Build history of the part. All positions in model axes, mm. Face numbers are marked on the shaded views. Round coordinates to 2 decimals unless told otherwise and drop trailing zeros. Loops run counter-clockwise (first coordinate to the right, second up) from the corner with the lowest first, then second, coordinate; pieces in that order, holes last. Notation, with made-up numbers: M -5,33 L 30,33 A24 ccw 30,62 Z; hole C 12.25,-28.5 d1. An arc over 180 degrees is marked long. Use one line per item in the form item = value. Start each with the question number.
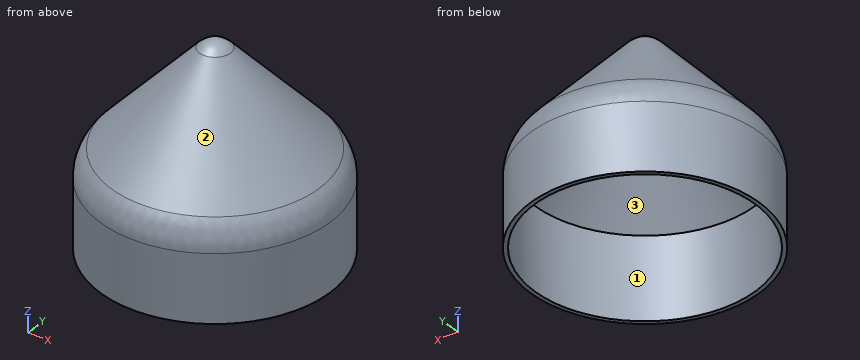
```python
from build123d import *

# Parameters (mm, degrees)
F0_W = 69.85
F0_H = 50.8
F2_T = -2.54
F3_R = 25.4


with BuildPart() as f1:
    # F0 (on Front) → F1 (revolve)
    with BuildSketch(Plane.XZ):
        with Locations((34.925, -25.4)):
            Rectangle(F0_W, F0_H)
        with BuildLine():
            Line((0, 70.105362), (0, 0))
            Line((0, 0), (69.85, 0))
            Line((69.85, 0), (9.361858, 65.987064))
            ThreePointArc((9.361858, 65.987064), (5.113823, 69.030284), (0, 70.105362))
        make_face()
    revolve(axis=Axis((0, 0, 38.1), (0, 0, 1)))

    # F2
    f2_openings = [f1.faces().sort_by_distance(p)[0] for p in [
        (0, 0, -50.8),
    ]]
    offset(amount=F2_T, openings=f2_openings)

    # F3
    f3_edges = [f1.edges().sort_by_distance(p)[0] for p in [
        (-69.85, 0, 0),
    ]]
    fillet(f3_edges, radius=F3_R)


solid = f1.part
```
Q1. Saw through at A-A (z = -32). Give the cut face in (x, y).
Q2. Saw through at B-B (z = 37). Give the cut face in (x, y), and give its area (3 significant figures).
Q3. Pull direction X, two halves, no side cores. Call the marked faces 1, 2 and 3: pulls with the +X half, pulls with the -X half, needs draft (parallel to the pull), parting line crosses it, or undercut.
Q4. Drop flat-ended pins along their axis: P1, Ø12, axis at y = -43.5, z = 8, coming from the +X side; P2, Ø1, axis at x = -27, z = -27.5, coming from the -Y side; P3, Ø12, axis at y = 6.5, z = 51, coming from the -X side. Give the stop position or say it passes through.
Q5. Wall check: probe 1 along Y at (x, z) = (0, -40); probe 2 along X at (y, z) = (15.5, 8); probe 3 along X at (y, z) = (-57, -25.5). Give the ranges that are in metal, low to high.
Filled in:
q1.outline = C 0,0 d139.7; hole C 0,0 d134.62
q2.outline = C 0,0 d71.87; hole C 0,0 d64.98
q2.area = 741 mm²
q3.face_1 = undercut
q3.face_2 = parting line crosses it
q3.face_3 = undercut
q4.P1 = 52.91
q4.P2 = -64.63
q4.P3 = -27.99
q5.probe_1 = -69.85 to -67.31, 67.31 to 69.85
q5.probe_2 = -60.56 to -57, 57 to 60.56
q5.probe_3 = -40.37 to -35.8, 35.8 to 40.37
